Part model, mm, in its own coordinate system. Give positions to 0.01 mm unless a question says otherwise; leave off trailing zeros. Write each loop counter-clockwise with the first axis right and the second up, starting at its lowest first coordinate (ties: lowest second). Pieces come first, ordered by that corner, then holes. Notation, with made-up numbers: (-16.5, 29.25) - (-8.5, 29.25) arc R21 cw to (-8.5, 53.25) - close; hole circle Ø1 at (89.25, 33). An arc over 180 degrees is marked (long way). Answer as a JSON object with one key per item and string values. Group by question number.
```python
from build123d import *

# Parameters (mm, degrees)
F0_R     = 80
F1_DEPTH = 200


with BuildPart() as f1:
    # F0 (on Top) → F1 (new body)
    with BuildSketch(Plane.XY):
        Circle(F0_R)
    extrude(amount=F1_DEPTH)


with BuildPart() as f2_1:
    # F2: copy of F1
    add(f1.part)


solid = f1.part
```
1) Probe line 1 (X direction, y = -11, z = 175); line 2 (Y direction, x = 70, z = 93.5). List the from-to ranges inside material, lowest first.
2) Band-saw the part on C-C (x = 34.5). List the corners of the cut face in (y, z), plus the area to 3 significant figures.
3) Band-saw the part on B-B (y = -45). List the corners of the cut face in (x, z).
4) Band-saw the part on A-A (z = 185.5). List the corners of the cut face in (x, y), plus the area to 3 significant figures.
5) Drop flat-ended pins along their axis: P1, Ø2, axis at x = 35.5, z = 54.5, coming from the +Y side; P2, Ø2, axis at y = 40.5, z = 174, coming from the -X side; P3, Ø4, axis at x = 43, z = 106.5, coming from the +Y side (3 decimals). Give the stop position or say it passes through.
Verdict:
{
 "1": {"line 1": "-79.24 to 79.24", "line 2": "-38.73 to 38.73"},
 "2": {"outline": "(-72.18, 0) - (72.18, 0) - (72.18, 200) - (-72.18, 200) - close", "area": "28,900 mm2"},
 "3": {"outline": "(-66.14, 0) - (66.14, 0) - (66.14, 200) - (-66.14, 200) - close"},
 "4": {"outline": "circle Ø160 at (0, 0)", "area": "20,100 mm2"},
 "5": {"P1": "y = 72.18", "P2": "x = -69.57", "P3": "y = 68.695"}
}
